from build123d import *

# Parameters (mm, degrees)
CYLINDER_R     = 9.7
CYLINDER_DEPTH = 50
TUBE_R         = 20
TUBE_R_2       = 7.5
TUBE_DEPTH     = 50


with BuildPart() as bearing_hole_cutter:
    # Cylinder → Cylinder (new body)
    with BuildSketch(Plane.XY.offset(14)):
        Circle(CYLINDER_R)
    extrude(amount=CYLINDER_DEPTH)


with BuildPart() as cut:
    # Tube → Tube (new body)
    with BuildSketch(Plane.XY):
        Circle(TUBE_R)
        Circle(TUBE_R_2, mode=Mode.SUBTRACT)
    extrude(amount=TUBE_DEPTH)

    # Cut: cut Bearing Hole cutter
    add(bearing_hole_cutter.part, mode=Mode.SUBTRACT)


solid = cut.part
Here's how the part is built. I have some questions about the finished solid (model axes, mm). A direction names the side the tool comes from. Round coordinates to 2 decimals unless told otherwise and drop trailing zeros. Loops run counter-clockwise (first coordinate to the right, second up) from the corner with the lowest first, then second, coordinate; pieces in that order, holes last.
1. If we section it at A-A on y = 0: Write out the boundary of the cut face in (x, z), plus the area to 3 significant figures.
Answer list:
outline: (-20, 0) - (-7.5, 0) - (-7.5, 14) - (-9.7, 14) - (-9.7, 50) - (-20, 50) - close; (7.5, 0) - (20, 0) - (20, 50) - (9.7, 50) - (9.7, 14) - (7.5, 14) - close
area: 1,090 mm2
2. Which directions (+Z, -Z, +X, -X, +Y, -Y) give clear straight access to the entire face, cutting with the end or side of a thin tool? Please do faces 4 (the face through (-5, -9, 50)), 5 (the face through (9.252, 2.914, 31.748)).
Answer list:
face 4: +Z, +X, -X, +Y, -Y
face 5: +Z
3. For P1, Ø3, axis at x = -1, z = 12.5, coming from the -Y side; P2, Ø3, axis at y = 10.5, z = 5, coming from the +X side; P3, Ø4, axis at x = -7.5, z = 39.5, coming from the +Y side, each with a flat end and sliding along its axis, tell me the tip position at first contact or that it passes through.
Answer list:
P1: stops at y = -20
P2: stops at x = 17.86
P3: stops at y = 19.23
4. If we section it at D-D on y = -8.5: Write out the boundary of the cut face in (x, z), plus the area to 3 significant figures.
Answer list:
outline: (-18.1, 0) - (18.1, 0) - (18.1, 50) - (4.67, 50) - (4.67, 14) - (-4.67, 14) - (-4.67, 50) - (-18.1, 50) - close
area: 1,470 mm2
5. We'd pull the mould along X, two halves only. Please class faces 1 (the face through (-7.493, 0.33, 6.902)), 2 (the face through (0, -9, 0)), 3 (the face through (-4.336, -19.524, 24.65)): +X half, -X half, draft (parallel to the pull), parting line (faces both ways), or undercut.
Answer list:
face 1: undercut
face 2: draft
face 3: parting line
6. If we section it at C-C on z = 5: Write out the boundary of the cut face in (x, y), plus the area to 3 significant figures.
Answer list:
outline: circle Ø40 at (0, 0); hole circle Ø15 at (0, 0)
area: 1,080 mm2
7. If I drill on line 1 along Y through (x, z) = (0, 3.5); line 2 along Y through (x, z) = (0, 24); line 3 along Z through (x, y) = (1.5, -8.5), over which ranges is the centre line in solid material (lowest first)?
Answer list:
line 1: y = -20 to -7.5, 7.5 to 20
line 2: y = -20 to -9.7, 9.7 to 20
line 3: z = 0 to 14
